Read the model definition and answer for the solid it produces. Units are mm, in the model's axes. A direction names the side the tool comes from. Give positions to 0.01 mm unless a question says otherwise; leave off trailing zeros. Order: outer loops, then holes, each group sorted by start corner. A loop starts at its lowest first (then second) coordinate and runs counter-clockwise, first axis right, second up.
Autodesk Inventor part; units mm, degrees
ref_plane "YZ Plane" through (0, 0, 0) normal (1, 0, 0) x (0, 1, 0)
ref_plane "XZ Plane" through (0, 0, 0) normal (0, 1, 0) x (-1, 0, 0)
ref_plane "XY Plane" through (0, 0, 0) normal (0, 0, 1) x (1, 0, 0)
sketch "Sketch1" plane through (0, 0, 0) normal (0, 0, 1) x (1, 0, 0)
  line L0 (-6.698639, 7.691729) -> (4.001361, 7.691729)
  line L1 (4.001361, 7.691729) -> (4.001361, -6.308271)
  line L2 (4.001361, -6.308271) -> (-6.698639, -6.308271)
  line L3 (-6.698639, -6.308271) -> (-6.698639, 7.691729)
  line L4 (4.001361, -6.308271) -> (-6.698639, -6.308271)
  line L5 (-6.698639, -6.308271) -> (-6.698639, -2.808271)
  line L6 (-6.698639, -2.808271) -> (4.001361, -2.808271)
  line L7 (4.001361, -2.808271) -> (4.001361, -6.308271)
  line L8 (-6.698639, -6.308271) -> (-5.698639, -6.308271)
  line L9 (-5.698639, -6.308271) -> (-5.698639, 7.691729)
  line L10 (-5.698639, 7.691729) -> (-6.698639, 7.691729)
  line L11 (-6.698639, 7.691729) -> (-6.698639, -6.308271)
  line L12 (-5.698639, -2.808271) -> (3.472299, -2.808271)
  line L13 (3.472299, -2.808271) -> (3.472299, -0.408271)
  line L14 (3.472299, -0.408271) -> (-5.698639, -0.408271)
  line L15 (-5.698639, -0.408271) -> (-5.698639, -2.808271)
  line L16 (-5.698639, -0.408271) -> (-1.298639, -0.408271)
  line L17 (-1.298639, -0.408271) -> (-1.298639, -2.808271)
  line L18 (-1.298639, -2.808271) -> (-5.698639, -2.808271)
  line L19 (-5.698639, -2.808271) -> (-5.698639, -0.408271)
  point P0 (0, 0)
  dimension "d0" = 10.7
  dimension "d1" = 14
  dimension "d2" = 3.5
  dimension "d3" = 1
  dimension "d4" = 2.4
  dimension "d5" = 4.4
extrude "Extrusion1" add sketch "Sketch1" against normal blind 1.6
extrude "Extrusion2" add sketch "Sketch1" along normal blind 1.1 contours L14 L17 L6 L9
sketch "Sketch2" plane through (0, 0, 0) normal (0, 0, 1) x (1, 0, 0)
  line L0 (-1.298639, -0.408271) -> (-1.298639, -2.808271)
  line L1 (-1.298639, -2.808271) -> (-5.698639, -2.808271)
  line L2 (-5.698639, -2.808271) -> (-5.698639, -0.408271)
  line L3 (-5.698639, -0.408271) -> (-1.298639, -0.408271)
  line L4 (4.001361, 7.691729) -> (-6.698639, 7.691729)
  line L5 (-6.698639, 7.691729) -> (-6.698639, -6.308271)
  line L6 (-6.698639, -6.308271) -> (4.001361, -6.308271)
  line L7 (4.001361, -6.308271) -> (4.001361, 7.691729)
  line L8 (4.001361, -6.308271) -> (4.001361, 7.691729)
  line L9 (-6.698639, 7.691729) -> (-6.698639, -6.308271)
  line L10 (4.001361, -6.308271) -> (-6.698639, -6.308271)
  line L11 (-6.698639, -6.308271) -> (-6.698639, -5.308271)
  line L12 (-6.698639, -5.308271) -> (4.001361, -5.308271)
  line L13 (4.001361, -5.308271) -> (4.001361, -6.308271)
  line L14 (4.001361, -6.308271) -> (3.001361, -6.308271)
  line L15 (3.001361, -6.308271) -> (3.001361, -2.808271)
  line L16 (3.001361, -2.808271) -> (4.001361, -2.808271)
  line L17 (4.001361, -2.808271) -> (4.001361, -6.308271)
  line L18 (-6.698639, -6.308271) -> (-0.098639, -6.308271)
  line L19 (-0.098639, -6.308271) -> (-0.098639, -2.808271)
  line L20 (-0.098639, -2.808271) -> (-6.698639, -2.808271)
  line L21 (-6.698639, -2.808271) -> (-6.698639, -6.308271)
  circle A0 centre (1.451361, -3.758271) radius 1.55
  point P0 (0, 0)
  dimension "d10" = 1
  dimension "d11" = 1
  dimension "d12" = 6.6
extrude "Extrusion3" cut sketch "Sketch2" against normal through all contours A0
sketch "Sketch3" plane through (0, 0, 0) normal (0, 0, 1) x (1, 0, 0)
  line L0 (4.001361, 7.691729) -> (4.001361, -6.308271)
  line L1 (-6.698639, 7.691729) -> (4.001361, 7.691729)
  line L2 (4.001361, 7.691729) -> (4.001361, 6.691729)
  line L3 (4.001361, 6.691729) -> (-6.698639, 6.691729)
  line L4 (-6.698639, 6.691729) -> (-6.698639, 7.691729)
  line L5 (-6.698639, 7.691729) -> (-5.698639, 7.691729)
  line L6 (-5.698639, 7.691729) -> (-5.698639, 5.612457)
  line L7 (-5.698639, 5.612457) -> (-6.698639, 5.612457)
  line L8 (-6.698639, 5.612457) -> (-6.698639, 7.691729)
  line L9 (-5.698639, 6.691729) -> (-4.598639, 6.691729)
  line L10 (-4.598639, 6.691729) -> (-4.598639, 6.161753)
  line L11 (-4.598639, 6.161753) -> (-5.698639, 6.161753)
  line L12 (-5.698639, 6.161753) -> (-5.698639, 6.691729)
  circle A0 centre (-5.148639, 6.141729) radius 0.55
  circle A1 centre (-2.608639, 6.141729) radius 0.55
  line L13 (-2.058639, 6.161753) -> (-3.158639, 6.161753)
  circle A2 centre (-0.068639, 6.141729) radius 0.55
  line L14 (0.481361, 6.161753) -> (-0.618639, 6.161753)
  circle A3 centre (2.471361, 6.141729) radius 0.55
  line L15 (3.021361, 6.161753) -> (1.921361, 6.161753)
  circle A4 centre (1.451361, -3.758271) radius 1.55
  line L16 (-1.298639, -0.408271) -> (-1.298639, -2.808271)
  line L17 (-1.298639, -2.808271) -> (-5.698639, -2.808271)
  line L18 (-5.698639, -2.808271) -> (-5.698639, -0.408271)
  line L19 (-5.698639, -0.408271) -> (-1.298639, -0.408271)
  line L20 (4.001361, 7.691729) -> (-6.698639, 7.691729)
  line L21 (-6.698639, 7.691729) -> (-6.698639, -6.308271)
  line L22 (-6.698639, -6.308271) -> (4.001361, -6.308271)
  line L23 (4.001361, -6.308271) -> (4.001361, 7.691729)
  line L24 (-6.698639, -6.308271) -> (-5.698639, -6.308271)
  line L25 (-5.698639, -6.308271) -> (-5.698639, -3.371834)
  line L26 (-5.698639, -3.371834) -> (-6.698639, -3.371834)
  line L27 (-6.698639, -3.371834) -> (-6.698639, -6.308271)
  line L28 (-6.698639, -6.308271) -> (4.001361, -6.308271)
  line L29 (-6.698639, -6.308271) -> (-3.498639, -6.308271)
  line L30 (-3.498639, -6.308271) -> (-3.498639, -5.308271)
  line L31 (-3.498639, -5.308271) -> (-6.698639, -5.308271)
  line L32 (-6.698639, -5.308271) -> (-6.698639, -6.308271)
  line L33 (-5.698639, -6.308271) -> (-4.598639, -6.308271)
  line L34 (-4.598639, -6.308271) -> (-4.598639, -3.371834)
  line L35 (-4.598639, -3.371834) -> (-5.698639, -3.371834)
  line L36 (-5.698639, -3.371834) -> (-5.698639, -6.308271)
  circle A5 centre (-5.148639, -4.758271) radius 0.55
  circle A6 centre (-2.608639, -4.758271) radius 0.55
  line L37 (-0.958639, -5.308271) -> (-4.158639, -5.308271)
  point P0 (0, 0)
  dimension "d15" = 1
  dimension "d16" = 1
  dimension "d17" = 1.1
  dimension "d20" = 2.54
  dimension "d25" = 1
  dimension "d26" = 1
  dimension "d27" = 1.1
  dimension "d30" = 2.54
sketch "Sketch3 outline for Extrusion4" plane through (0, 0, 0) normal (0, 0, 1) x (1, 0, 0)
  circle A0 centre (-5.148639, -4.758271) radius 0.55
  circle A1 centre (-2.608639, -4.758271) radius 0.55
  circle A2 centre (2.471361, 6.141729) radius 0.55
  circle A3 centre (-0.068639, 6.141729) radius 0.55
  circle A4 centre (-2.608639, 6.141729) radius 0.55
  circle A5 centre (-5.148639, 6.141729) radius 0.55
extrude "Extrusion4" cut sketch "Sketch3 outline for Extrusion4" against normal through all
sketch "Sketch4" plane through (-5.698639, -0.408271, 0) normal (0, 1, 0) x (1, 0, 0)
  line L0 (0, 0) -> (4.4, 0)
  line L1 (0, 0) -> (0, -1.1)
  line L2 (4.4, -1.1) -> (0, -1.1)
  line L3 (4.4, 0) -> (4.4, -1.1)
  line L4 (0, -1.1) -> (-17.024616, -77.893079)
  line L5 (4.4, -1.1) -> (11.53177, -33.269335)
  line L6 (2.2, -1.1) -> (2.2, -23.383849)
  line L7 (4.4, -1.1) -> (0, -1.1)
  line L8 (11.53177, -33.269335) -> (26.881941, -102.509481)
  circle A0 centre (2.2, -1.1) radius 22.283849
  line L9 (2.2, -23.383849) -> (9.005719, -21.875057)
  line L10 (2.2, -23.383849) -> (-4.605719, -21.875057)
  point P0 (5.698639, 0)
  dimension "d37" = 12.5
  dimension "d38" = 12.5
extrude "Wyciągnięcie proste5" add sketch "Sketch4" against normal blind 1 contours L2 L6 L10 L4 | L5 L9 L6 L2
sketch "Szkic5" plane through (-5.698639, -0.408271, 0) normal (0, 1, 0) x (1, 0, 0)
  line L0 (0, 0) -> (4.4, 0)
  line L1 (0, 0) -> (0, -1.1)
  line L2 (0, -1.1) -> (-4.605719, -21.875057)
  line L3 (-4.605719, -21.875057) -> (2.2, -23.383849)
  line L4 (2.2, -23.383849) -> (9.005719, -21.875057)
  line L5 (9.005719, -21.875057) -> (4.4, -1.1)
  line L6 (4.4, 0) -> (4.4, -1.1)
  line L7 (0, -1.1) -> (4.4, -1.1)
  line L8 (4.4, -1.1) -> (26.847507, -102.354162)
  line L9 (2.2, -1.1) -> (2.2, -251.1)
  line L10 (26.847507, -102.354162) -> (58.457755, -244.938774)
  line L11 (0, -1.1) -> (-54.057755, -244.938774)
  line L12 (2.2, -1.1) -> (2.2, 19.845326)
  line L13 (0, -1.1) -> (4.4, 18.747117)
  arc A0 (-54.057755, -244.938774) -> (58.457755, -244.938774) centre (2.2, 8.823559) ccw
  line L14 (2.2, -251.1) -> (0, -251.1)
  point P0 (5.698639, 0)
  dimension "d41" = 250
sketch "Szkic6" plane through (-5.698639, -0.408271, 0) normal (0, 1, 0) x (1, 0, 0)
  line L0 (2.2, -23.383849) -> (-4.605719, -21.875057)
  line L1 (-4.605719, -21.875057) -> (2.53543, 10.336584)
  line L2 (9.005719, -21.875057) -> (2.2, -23.383849)
  line L3 (9.005719, -21.875057) -> (2.2, 8.823559)
  line L4 (2.2, 8.823559) -> (2.2, -23.383849)
  line L5 (2.2, 8.823559) -> (-2.082149, -26.051744)
  line L6 (2.2, 8.823559) -> (6.293179, -24.512711)
  point P0 (5.698639, 0)
  dimension "d42" = 7
  dimension "d43" = 7
properties part number "TOF_VLCOS"
1) Given pin 1 (0.8 mm diameter, centred on y = -2.5, z = -0.5, fed in from -X); pin 2 (1.4 mm diameter, centred on x = -2.61, y = -4.76, fed in from +Z); pin 3 (1 mm diameter, centred on x = -3, z = 14.5, fed in from +Y), each flat-ended and moving along its own axis, determine where each tip first touches the part or whether it passes through.
Final values:
pin 1: stops at x = -6.7
pin 2: stops at z = 0
pin 3: stops at y = -0.41
2) The part is cut by section A-A on x = 1.25. Determine the outline of the cut face in (y, z), and give its area (3 significant figures).
Final values:
outline: (-6.31, -1.6) - (-5.3, -1.6) - (-5.3, 0) - (-6.31, 0) - close; (-2.22, -1.6) - (7.69, -1.6) - (7.69, 0) - (-2.22, 0) - close; (-1.41, 12.6) - (-0.41, 12.6) - (-0.41, 22.33) - (-1.41, 22.33) - close
area: 27.2 mm2
3) The part is cut by section C-C on y = 0. Determine the outline of the cut face in (x, z), and give its area (3 significant figures).
Final values:
outline: (-6.7, -1.6) - (4, -1.6) - (4, 0) - (-6.7, 0) - close
area: 17.1 mm2
4) The part is cut by section D-D on z = 3. Determine the outline of the cut face in (x, y), and give its area (3 significant figures).
Final values:
outline: (-6.12, -1.41) - (-0.88, -1.41) - (-0.88, -0.41) - (-6.12, -0.41) - close
area: 5.24 mm2
5) For a pull along X with two mould halves and no side action, classify faces 5 (the face through (-6.85, -0.9, 22.64)), 6 (the face through (-2.1, 5.93, -0.79)), 7 (the face through (-3.5, -2.808, 0.5)) as released by +X, released by -X, zero draft, split by the parting line, or undercut.
Final values:
face 5: released by -X
face 6: undercut
face 7: zero draft
6) A tool of negligible diameter and unlimited length cuts with its end or side. For faces 1 (the face through (-3, -0.408, 14)), 2 (the face through (-1.299, -1.6, 0.5)), 3 (the face through (-4, -2, 1.1)), 4 (the face through (-5.699, -1.6, 0.5)), from which of +Z, -Z, +X, -X, +Y, -Y can it reach the whole face along a straight path? Write none if from no direction.
Final values:
face 1: +Z, +X, -X, +Y
face 2: +X, +Y, -Y
face 3: +Z, +X, -X, -Y
face 4: -X, +Y, -Y
7) The part is cut by section B-B on x = -5.25. Determine the outline of the cut face in (y, z), and give its area (3 significant figures).
Final values:
outline: (-6.31, -1.6) - (-5.3, -1.6) - (-5.3, 0) - (-6.31, 0) - close; (-4.22, -1.6) - (5.6, -1.6) - (5.6, 0) - (-0.41, 0) - (-0.41, 23) - (-1.41, 23) - (-1.41, 1.1) - (-2.81, 1.1) - (-2.81, 0) - (-4.22, 0) - close; (6.68, -1.6) - (7.69, -1.6) - (7.69, 0) - (6.68, 0) - close
area: 43.5 mm2
8) Consider L1, parallel to Z at x = 2.5, y = 2.5; L2, parallel to Y at x = -6, z = 20; L3, parallel to X at y = -0.75, z = 10.75. Determine where each line is inside the solid, lowest interval first.
Final values:
L1: z = -1.6 to 0
L2: y = -1.41 to -0.41
L3: x = -7.84 to 0.84
